Verification items for the finished model (mm, model axes). A direction names the side the tool comes from. Coordinates: 2 decimals unless noted, no trailing zeros. Write each loop counter-clockwise with the first axis right and the second up, starting at its lowest first coordinate (ties: lowest second). Pieces come first, ordered by that corner, then holes. Notation, with made-up numbers: (-16, 30.25) -> (43, 30.25) arc R21 cw to (43, 64.25) -> close; hole circle Ø7 at (35.25, 70.5). An arc over 180 degrees is marked (long way). Write item = value, one per line. Start each with the question number.
(1) Section check B-B (z = 0). Record the cut outline in (x, y).
(2) Set-up check for faces 1 (the face through (53, 4, -4)), 2 (the face through (19, 23, 15)), 3 (the face through (34.032, 5.265, -0.21)): record each of +Z, -Z, +X, -X, +Y, -Y from which the full face is reachable in a straight line by a thin tool's end or side.
(3) Gauge pin test, flat ends, axial feed: pin 1 Ø4 at (x, y) = (28, 20) entering from -Z; pin 2 Ø5.5 at (y, z) = (51.5, 5) entering from +X; pin 3 Ø10 at (x, z) = (51, 1) entering from +Y; pin 4 Ø12 at (x, z) = (28, 6.5) entering from +Y. Record the tip position at first contact, or that the pin passes through.
(4) Mould release check, pull along X, two halves, no side actions. Record for faces 4 (the face through (24, 4, 0)), 5 (the face through (2.03, 54.39, -0.98)), 6 (the face through (23, 23, 0)): released by +X, released by -X, zero draft, split by the parting line, or undercut.
(5) Material ranges on probe 1 along Y at (x, z) = (1.45, 0); probe 2 along Y at (x, z) = (8, 4), recorded low to high. Write a range as [from, to].
(6) Section check A-A (y = 50). Record the cut outline in (x, z), plus the area to 3 significant figures.
(7) Section check D-D (z = -7.5). Record the cut outline in (x, y), plus the area to 3 significant figures.
Autodesk Inventor part; units mm, degrees
ref_plane "cover_panel_hole_a_XY" through (8, 8, 15) normal (0, 0, 1) x (1, 0, 0)
ref_plane "cover_panel_hole_a_YZ" through (8, 8, 15) normal (1, 0, 0) x (0, 1, 0)
ref_plane "cover_panel_hole_a_ZX" through (8, 8, 15) normal (0, 1, 0) x (0, 0, 1)
sketch "Skizze_1" plane through (0, 0, 0) normal (0, 0, 1) x (1, 0, 0)
  line L0 (0, 0) -> (60, 0)
  line L1 (60, 0) -> (60, 4)
  line L2 (60, 4) -> (42, 4)
  line L3 (42, 4) -> (4, 42)
  line L4 (4, 42) -> (4, 60)
  line L5 (4, 60) -> (0, 60)
  line L6 (0, 60) -> (0, 0)
extrude "Extrusion1" add sketch "Skizze_1" along normal mid plane 30
sketch "Skizze_2" plane through (0, 0, 0) normal (0, 0, 1) x (1, 0, 0)
  arc A0 (4, 17) -> (8, 13) centre (8, 17) ccw
  line L0 (8, 13) -> (9, 13)
  arc A1 (13, 9) -> (9, 13) centre (9, 9) ccw
  line L1 (13, 9) -> (13, 8)
  arc A2 (13, 8) -> (17, 4) centre (17, 8) ccw
  line L2 (17, 4) -> (32.1716, 4)
  arc A3 (32.1716, 4) -> (33.5858, 7.4142) centre (32.1716, 6) ccw
  line L3 (33.5858, 7.4142) -> (7.4142, 33.5858)
  arc A4 (7.4142, 33.5858) -> (4, 32.1716) centre (6, 32.1716) ccw
  line L4 (4, 32.1716) -> (4, 17)
extrude "Extrusion2" cut sketch "Skizze_2" along normal mid plane 32
sketch "Skizze_3" plane through (0, 0, 0) normal (0, 0, 1) x (1, 0, 0)
  circle A0 centre (8, 8) radius 2.5
extrude "Extrusion3" cut sketch "Skizze_3" along normal mid plane 32
sketch "Sketch4" plane through (0, 0, 15) normal (0, -1, 0) x (1, 0, 0)
  point P0 (50, -15)
hole "Drilling 2" at (50, 0, 0) direction (0, 1, 0) diameter 9 depth 5
sketch "Sketch5" plane through (0, 0, 15) normal (-1, 0, 0) x (0, 0, 1)
  point P0 (-15, 50)
hole "Drilling 3" at (0, 50, 0) direction (1, 0, 0) diameter 9 depth 5
ref_plane "cover_panel_hole_a_XY" through (8, 8, 15) normal (0, 0, 1) x (1, 0, 0)
ref_plane "cover_panel_hole_a_YZ" through (8, 8, 15) normal (1, 0, 0) x (0, 1, 0)
ref_plane "cover_panel_hole_a_ZX" through (8, 8, 15) normal (0, 1, 0) x (0, 0, 1)
ref_plane "cover_panel_hole_b_XY" through (8, 8, -15) normal (0, 0, -1) x (1, 0, 0)
ref_plane "cover_panel_hole_b_YZ" through (8, 8, -15) normal (1, 0, 0) x (0, -1, 0)
ref_plane "cover_panel_hole_b_ZX" through (8, 8, -15) normal (0, -1, 0) x (0, 0, -1)
ref_plane "side_1_XY" through (0, 30, 0) normal (-1, 0, 0) x (0, 0, 1)
ref_plane "side_1_YZ" through (0, 30, 0) normal (0, 0, 1) x (0, 1, 0)
ref_plane "side_1_ZX" through (0, 30, 0) normal (0, 1, 0) x (-1, 0, 0)
ref_plane "side_2_XY" through (30, 0, 0) normal (0, -1, 0) x (0, 0, 1)
ref_plane "side_2_YZ" through (30, 0, 0) normal (0, 0, 1) x (-1, 0, 0)
ref_plane "side_2_ZX" through (30, 0, 0) normal (-1, 0, 0) x (0, -1, 0)
properties part number "MayTec 1.46.20639_Angle Alu 60x60, D9.0, B30"
Response:
q1.outline = (0, 0) -> (45.5, 0) -> (45.5, 4) -> (42, 4) -> (4, 42) -> (4, 45.5) -> (0, 45.5) -> close; (0, 54.5) -> (4, 54.5) -> (4, 60) -> (0, 60) -> close; (54.5, 0) -> (60, 0) -> (60, 4) -> (54.5, 4) -> close; hole (4, 17) arc R4 ccw to (8, 13) -> (9, 13) arc R4 cw to (13, 9) -> (13, 8) arc R4 ccw to (17, 4) -> (32.17, 4) arc R2 ccw to (33.59, 7.41) -> (7.41, 33.59) arc R2 ccw to (4, 32.17) -> close; hole circle Ø5 at (8, 8)
q2.face_1 = +Z, -Z, +X, +Y
q2.face_2 = +Z, +X, -X, +Y, -Y
q2.face_3 = +Z, -Z
q3.pin_1 = -15
q3.pin_2 = 4
q3.pin_3 = 4
q3.pin_4 = 24
q4.face_4 = undercut
q4.face_5 = zero draft
q4.face_6 = released by +X
q5.probe_1 = [0, 45.5], [54.5, 60]
q5.probe_2 = [0, 5.5], [10.5, 13], [33, 38]
q6.outline = (0, -15) -> (4, -15) -> (4, -4.5) -> (0, -4.5) -> close; (0, 4.5) -> (4, 4.5) -> (4, 15) -> (0, 15) -> close
q6.area = 84.0 mm2
q7.outline = (0, 0) -> (60, 0) -> (60, 4) -> (42, 4) -> (4, 42) -> (4, 60) -> (0, 60) -> close; hole (4, 17) arc R4 ccw to (8, 13) -> (9, 13) arc R4 cw to (13, 9) -> (13, 8) arc R4 ccw to (17, 4) -> (32.17, 4) arc R2 ccw to (33.59, 7.41) -> (7.41, 33.59) arc R2 ccw to (4, 32.17) -> close; hole circle Ø5 at (8, 8)
q7.area = 716 mm2
